CAD build for the part. Positions are in the model's coordinates, mm. Give positions to 0.01 mm unless a question says otherwise; leave off trailing zeros. Write each loop counter-clockwise with the first axis right and the second up, starting at its lowest first coordinate (ties: lowest second). Pieces come first, ordered by that corner, then holes. Notation, with made-up numbers: (84, 44.25) - (112, 44.25) arc R24 ccw to (112, 62.25) - close; hole circle Ø2 at (5.5, -30.75). An arc over 180 degrees is marked (long way). Put each result on its own line as item: value. Start each with the question number.
1. Cut at C-C on z = 2.05. List the corners of the cut face in (x, y), and give its area (3 significant figures).
2. Cut at D-D on y = 10. List the corners of the cut face in (x, z), and give its area (3 significant figures).
3. Cut at B-B on y = 4. List the corners of the cut face in (x, z), and give its area (3 significant figures).
4. Cut at A-A on x = 25. List the corners of the cut face in (y, z).
5. Wall check: line 1 (X direction, y = 0.5, z = 2.3); line 2 (Y direction, x = 25, z = 1.55); line 3 (X direction, y = 9.5, z = 0.5). Give the ranges that are in metal, low to high.
6. Drop flat-ended pins along their axis: pin 1 (1.5 mm diameter, centred on y = -11, z = 0.5, fed in from -X); pin 2 (10 mm diameter, centred on x = -9, y = -0.5, fed in from +Z); pin 3 (1.5 mm diameter, centred on x = 7, z = 1, fed in from +Y); pin 4 (1.5 mm diameter, centred on y = 4.5, z = 2.5, fed in from -X). Give the stop position or say it passes through.
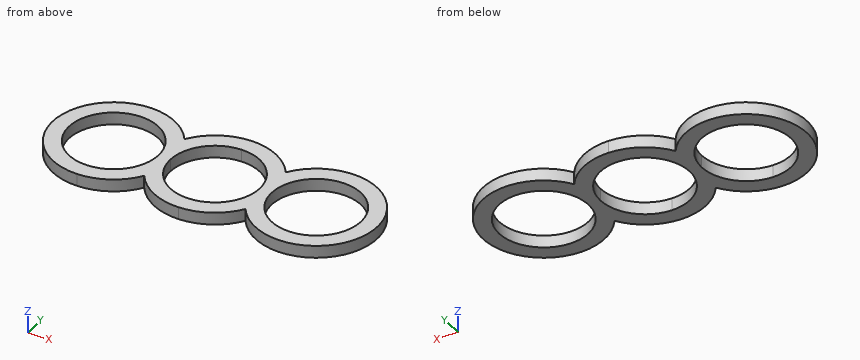
from build123d import *

# Parameters (mm, degrees)
F1_DEPTH = 3


with BuildPart() as f1:
    # F0 (on Top) → F1 (new body)
    with BuildSketch(Plane.XY):
        with BuildLine():
            ThreePointArc((-25, -15), (-17.9068141727, -13.2169101843), (-12.5, -8.2915619759))
            ThreePointArc((-12.5, -8.2915619759), (-7.0931858273, -13.2169101843), (0, -15))
            ThreePointArc((0, -15), (7.0931858273, -13.2169101843), (12.5, -8.2915619759))
            ThreePointArc((12.5, -8.2915619759), (40, 0), (12.5, 8.2915619759))
            ThreePointArc((12.5, 8.2915619759), (7.0931858273, 13.2169101843), (0, 15))
            ThreePointArc((0, 15), (-7.0931858273, 13.2169101843), (-12.5, 8.2915619759))
            ThreePointArc((-12.5, 8.2915619759), (-38.2169101843, 7.0931858273), (-25, -15))
        make_face()
        with BuildLine():
            ThreePointArc((-14, 0), (-17.2218254069, -7.7781745931), (-25, -11))
            ThreePointArc((-25, -11), (-32.7781745931, 7.7781745931), (-14, 0))
        make_face(mode=Mode.SUBTRACT)
        with BuildLine():
            ThreePointArc((-11, 0), (-7.7781745931, 7.7781745931), (0, 11))
            ThreePointArc((0, 11), (7.7781745931, 7.7781745931), (11, 0))
            ThreePointArc((11, 0), (7.7781745931, -7.7781745931), (0, -11))
            ThreePointArc((0, -11), (-7.7781745931, -7.7781745931), (-11, 0))
        make_face(mode=Mode.SUBTRACT)
        with BuildLine():
            ThreePointArc((14, 0), (25, 11), (36, 0))
            ThreePointArc((36, 0), (25, -11), (14, 0))
        make_face(mode=Mode.SUBTRACT)
    extrude(amount=F1_DEPTH)


solid = f1.part
Report:
1. outline: (-12.5, -8.29) arc R15 ccw to (12.5, -8.29) arc R15 ccw (long way) to (12.5, 8.29) arc R15 ccw to (-12.5, 8.29) arc R15 ccw (long way) to start; hole circle Ø22 at (-25, 0); hole circle Ø22 at (0, 0); hole circle Ø22 at (25, 0)
1. area: 868 mm²
2. outline: (-36.18, 0) - (-29.58, 0) - (-29.58, 3) - (-36.18, 3) - close; (-20.42, 0) - (-13.82, 0) - (-13.82, 3) - (-20.42, 3) - close; (-11.18, 0) - (-4.58, 0) - (-4.58, 3) - (-11.18, 3) - close; (4.58, 0) - (11.18, 0) - (11.18, 3) - (4.58, 3) - close; (13.82, 0) - (20.42, 0) - (20.42, 3) - (13.82, 3) - close; (29.58, 0) - (36.18, 0) - (36.18, 3) - (29.58, 3) - close
2. area: 119 mm²
3. outline: (-39.46, 0) - (-35.25, 0) - (-35.25, 3) - (-39.46, 3) - close; (-14.75, 0) - (-10.25, 0) - (-10.25, 3) - (-14.75, 3) - close; (10.25, 0) - (14.75, 0) - (14.75, 3) - (10.25, 3) - close; (35.25, 0) - (39.46, 0) - (39.46, 3) - (35.25, 3) - close
3. area: 52.3 mm²
4. outline: (-15, 0) - (-11, 0) - (-11, 3) - (-15, 3) - close; (11, 0) - (15, 0) - (15, 3) - (11, 3) - close
5. line 1: x = -39.99 to -35.99, -14.01 to -10.99, 10.99 to 14.01, 35.99 to 39.99
5. line 2: y = -15 to -11, 11 to 15
5. line 3: x = -36.61 to -30.55, -19.45 to -13.39, -11.61 to -5.55, 5.55 to 11.61, 13.39 to 19.45, 30.55 to 36.61
6. pin 1: stops at x = -35.95
6. pin 2: stops at z = 3
6. pin 3: stops at y = 13.64
6. pin 4: stops at x = -39.52
